from build123d import *

# Parameters (mm, degrees)
BOSS_EXTRU_1_DEPTH = 12.5
ESQUISSE2_R        = 2.5
BOSS_EXTRU_2_DEPTH = 2
ESQUISSE3_R        = 1
BOSS_EXTRU_3_DEPTH = 40


with BuildPart() as part:
    # Esquisse1 → Boss.-Extru.1 (new, symmetric)
    with BuildSketch(Plane.XY):
        with BuildLine():
            Line((-6.614378278, 7.5), (6.614378278, 7.5))
            ThreePointArc((6.614378278, 7.5), (10, 0), (6.614378278, -7.5))
            Line((6.614378278, -7.5), (-6.614378278, -7.5))
            ThreePointArc((-6.614378278, -7.5), (-10, 0), (-6.614378278, 7.5))
        make_face()
    extrude(amount=BOSS_EXTRU_1_DEPTH, both=True)

    # Esquisse2 → Boss.-Extru.2 (add)
    with BuildSketch(Plane.XY.offset(12.5)):
        Circle(ESQUISSE2_R)
    extrude(amount=BOSS_EXTRU_2_DEPTH)

    # Esquisse3 → Boss.-Extru.3 (add)
    with BuildSketch(Plane.XY.offset(14.5)):
        Circle(ESQUISSE3_R)
    extrude(amount=BOSS_EXTRU_3_DEPTH)


solid = part.part
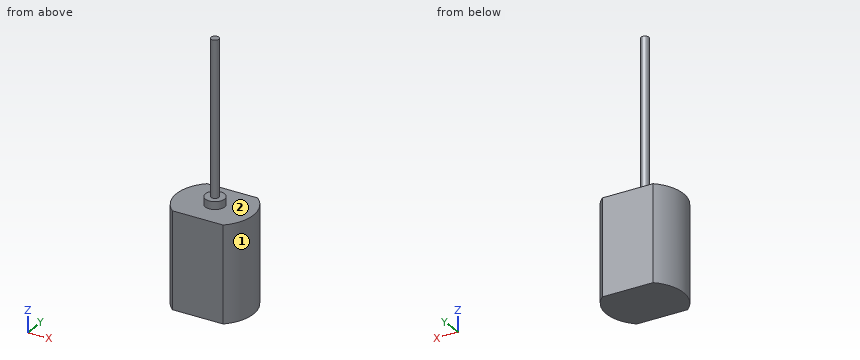
Build history of the part. All positions in model axes, mm. Face numbers are marked on the shaded views. A direction names the side the tool comes from. Round coordinates to 2 decimals unless told otherwise and drop trailing zeros. Write each loop counter-clockwise with the first axis right and the second up, starting at its lowest first coordinate (ties: lowest second). Pieces come first, ordered by that corner, then holes. Notation, with made-up numbers: M -18,59 L 12,59 A20 ccw 12,83 Z; hole C 24.5,63 d8. An arc over 180 degrees is marked long. Use CSV: the item, a comma, the result in double quotes.
1. Flat gauge pins, fed straight in: pin 1 (2 mm diameter, centred on y = 4.5, z = -3.5, fed in from -X); pin 2 (3 mm diameter, centred on x = 0.5, z = 32.5, fed in from -Y); pin 3 (2 mm diameter, centred on x = -7, y = -1.5, fed in from +Z). Where does each tip first touch, or does it go through?
Reply:
pin 1,"stops at x = -9.37"
pin 2,"stops at y = -1"
pin 3,"stops at z = 12.5"
2. Tool access for the marked faces 1 and 2: list every direction of +Z, -Z, +X, -X, +Y, -Y with a clear straight run to the whole face (end or side of a thin tool).
Reply:
face 1,"+Z, -Z, +X"
face 2,"+Z"
3. Saw through at B-B (x = 0). Give the cut face in (y, z), plus the area to 3 significant figures.
Reply:
outline,"M -7.5,-12.5 L 7.5,-12.5 L 7.5,12.5 L 2.5,12.5 L 2.5,14.5 L 1,14.5 L 1,54.5 L -1,54.5 L -1,14.5 L -2.5,14.5 L -2.5,12.5 L -7.5,12.5 Z"
area,"465 mm²"
4. Saw through at D-D (x = 8). Give the cut face in (y, z).
Reply:
outline,"M -6,-12.5 L 6,-12.5 L 6,12.5 L -6,12.5 Z"
5. Saw through at A-A (y = 0). Give the cut face in (x, z), plus the area to 3 significant figures.
Reply:
outline,"M -10,-12.5 L 10,-12.5 L 10,12.5 L 2.5,12.5 L 2.5,14.5 L 1,14.5 L 1,54.5 L -1,54.5 L -1,14.5 L -2.5,14.5 L -2.5,12.5 L -10,12.5 Z"
area,"590 mm²"
6. Wall check: probe 1 along Z at (x, y) = (-3, 0.5); probe 2 along Y at (x, z) = (-7.5, 9); probe 3 along Z at (x, y) = (-1, -0.25). Give the ranges that are in metal, low to high. Write a range as from..to.
Reply:
probe 1,"z = -12.5..12.5"
probe 2,"y = -6.61..6.61"
probe 3,"z = -12.5..14.5"
7. Saw through at C-C (z = 7). Give the cut face in (x, y).
Reply:
outline,"M -6.61,-7.5 L 6.61,-7.5 A10 ccw 6.61,7.5 L -6.61,7.5 A10 ccw Z"
